```python
from build123d import *

# Parameters (mm, degrees)
F0_W     = 20
F0_H     = 40
F0_W_2   = 16
F0_H_2   = 36
F1_DEPTH = 500
F2_R     = 4.5
F2_R_2   = 8
F3_DEPTH = 25


with BuildPart() as f1:
    # F0 (on Front) → F1 (new body)
    with BuildSketch(Plane.XZ):
        with Locations((10, -20)):
            Rectangle(F0_W, F0_H)
        with Locations((10, -20)):
            Rectangle(F0_W_2, F0_H_2, mode=Mode.SUBTRACT)
    extrude(amount=F1_DEPTH)

    # F2 (on face) → F3 (cut)
    with BuildSketch(Plane(origin=(0, 0, 0), x_dir=(0, -1, 0), z_dir=(-1, 0, 0))):
        with Locations((487.16492, -29.815726)):
            Circle(F2_R)
        with Locations((441.037512, -21.502786)):
            Circle(F2_R_2)
    extrude(amount=-F3_DEPTH, mode=Mode.SUBTRACT)


solid = f1.part
```
The listing builds one solid part. Answer for the finished solid, in the listing's coordinates (mm). A direction names the side the tool comes from. Coordinates: 2 decimals unless noted, no trailing zeros. Write each loop counter-clockwise with the first axis right and the second up, starting at its lowest first coordinate (ties: lowest second). Pieces come first, ordered by that corner, then holes. Notation, with made-up numbers: (-30, -27.75) - (18, -27.75) arc R10 cw to (18, -20.75) - close; hole circle Ø7 at (-29, -26). An arc over 180 degrees is marked (long way). One line per item, written item: value.
1) Find section A-A (z = -7.5). Give the vertices of the cut face in (x, y).
Geometry check:
outline: (0, -500) - (2, -500) - (2, 0) - (0, 0) - close; (18, -500) - (20, -500) - (20, 0) - (18, 0) - close
2) A tool of negligible diameter and unlimited length cuts with its end or side. For faces 1 (the flat face through (10, -246, 0)), 2 (the flat face through (10, -246, -38)), from which of +Z, -Z, +X, -X, +Y, -Y can it reach the whole face along a straight path? Write none if from no direction.
Geometry check:
face 1: +Z, +X, -X, +Y, -Y
face 2: +Y, -Y
3) Find section C-C (x = 6.5). Give the vertices of the cut face in (y, z).
Geometry check:
outline: (-500, -40) - (0, -40) - (0, -38) - (-500, -38) - close; (-500, -2) - (0, -2) - (0, 0) - (-500, 0) - close
4) Consider line 1 along X through (y, z) = (-339, -36.5); line 2 along Z through (x, y) = (14.5, -86). Determine where each line is inside the solid, lowest interval first. Write a range as from..to.
Geometry check:
line 1: x = 0..2, 18..20
line 2: z = -40..-38, -2..0
5) Find section B-B (y = -30.5). Give the vertices of the cut face in (x, z).
Geometry check:
outline: (0, -40) - (20, -40) - (20, 0) - (0, 0) - close; hole (2, -38) - (18, -38) - (18, -2) - (2, -2) - close
6) For a pull along Z with two mould halves and no side action, classify faces 3 (the flat face through (0, -246, -20)), 4 (the flat face through (10, -246, -40)), 5 (the cylindrical face through (0.99, -439.3, -29.31)), 6 (the flat face through (10, -246, -2)) as pulls with the +Z half, pulls with the -Z half, needs draft (parallel to the pull), parting line crosses it, or undercut.
Geometry check:
face 3: needs draft
face 4: pulls with the -Z half
face 5: undercut
face 6: undercut
